Design review of the part built by this model. Coordinates are the model's own, in mm. A direction names the side the tool comes from. Give positions to 0.01 mm unless a question says otherwise; leave off trailing zeros. Write each loop counter-clockwise with the first axis right and the second up, starting at its lowest first coordinate (ties: lowest second). Pieces come first, ordered by that corner, then holes. Notation, with made-up numbers: (83, 62) -> (96, 62) arc R20 ccw to (96, 98) -> close; hole circle Ø7 at (20, -7). An arc over 180 degrees is marked (long way). Write each question's results on one line, items separated by ' | '. Start each with the question number.
(1) For faces 4 (the face through (25.186, -1.915, -4.619)), 5 (the face through (-7, 19, 10)), list the 3-axis set-ups (+Z, -Z, +X, -X, +Y, -Y) from which the entire face can be reached by the end or side of a thin tool; tool diameter is ignored.
(2) Take a section at A-A (x = 0). State the section outline as (y, z) points, plus the area to 3 significant figures.
(3) Mouldability with a two-part tool opening along Y and no side actions: class faces 1 (the face through (-4.336, -19.524, -0.14)), 2 (the face through (-2.994, 22.804, 0.14)), 3 (the face through (28, 0, 0)) as released by +Y, released by -Y, zero draft, split by the parting line, or undercut.
(4) Clearance check with flat-ended pins moving along their axes: pin 1 (3 mm diameter, centred on y = 17.5, z = 4, fed in from -X); pin 2 (5 mm diameter, centred on x = 1, z = 3.5, fed in from +Y); pin 3 (2 mm diameter, centred on x = -18, z = -4, fed in from +Y). State where each tip first meets the part, or that it passes through.
(5) Take a section at B-B (y = 0). State the section outline as (x, z) points.
(6) To check wall thickness, follow probe 1 along Y at (x, z) = (0, -1.5); probe 2 along X at (y, z) = (5.5, -5.25); probe 3 along X at (y, z) = (-7.5, -8). State the ranges of each line that lie inside material, in increasing order.
(7) Take a section at C-C (z = 0). State the section outline as (x, y) points, plus the area to 3 significant figures.
(8) Take a section at D-D (x = 8). State the section outline as (y, z) points, plus the area to 3 significant figures.
from build123d import *

# Parameters (mm, degrees)
ESQUISSE1_R                    = 23
ESQUISSE1_R_2                  = 20
BOSS_EXTRU_1_DEPTH             = 10
BOSS_EXTRU_2_REACH             = 48
ESQUISSE2_R                    = 5
BOSS_EXTRU_2_DIRECTION_2_DEPTH = 5


with BuildPart() as part:
    # Esquisse1 → Boss.-Extru.1 (new body, symmetric)
    with BuildSketch(Plane.XY):
        Circle(ESQUISSE1_R)
        Circle(ESQUISSE1_R_2, mode=Mode.SUBTRACT)
    extrude(amount=BOSS_EXTRU_1_DEPTH, both=True)

    # Esquisse2 → Boss.-Extru.2 (add, up to next)
    with BuildSketch(Plane(origin=(23, 0, 0), x_dir=(0, 0, -1), z_dir=(1, 0, 0)), mode=Mode.PRIVATE) as boss_extru_2_sk1:
        Circle(ESQUISSE2_R)
    boss_extru_2_tool1 = extrude(boss_extru_2_sk1.sketch, amount=-BOSS_EXTRU_2_REACH, mode=Mode.PRIVATE) - part.part
    add(boss_extru_2_tool1.solids().sort_by_distance((23, 0, 0))[0])
    add(boss_extru_2_tool1.solids().sort_by_distance((23, 0, 0))[1])

    # Esquisse2 → Boss.-Extru.2 direction 2 (add)
    with BuildSketch(Plane(origin=(23, 0, 0), x_dir=(0, 0, -1), z_dir=(1, 0, 0))):
        Circle(ESQUISSE2_R)
    extrude(amount=BOSS_EXTRU_2_DIRECTION_2_DEPTH)


solid = part.part
Report:
1) face 4: +X | face 5: +Z, +X, -X, +Y, -Y
2) outline: (-23, -10) -> (-20, -10) -> (-20, 10) -> (-23, 10) -> close; (20, -10) -> (23, -10) -> (23, 10) -> (20, 10) -> close | area: 120 mm2
3) face 1: undercut | face 2: split by the parting line | face 3: zero draft
4) pin 1: x = -16.52 | pin 2: y = 23 | pin 3: y = 15.49
5) outline: (-23, -10) -> (-20, -10) -> (-20, 10) -> (-23, 10) -> close; (20, -10) -> (23, -10) -> (23, -5) -> (28, -5) -> (28, 5) -> (23, 5) -> (23, 10) -> (20, 10) -> close
6) probe 1: -23 to -20, 20 to 23 | probe 2: -22.33 to -19.23, 19.23 to 22.33 | probe 3: -21.74 to -18.54, 18.54 to 21.74
7) outline: (22.45, -5) -> (28, -5) -> (28, 5) -> (22.45, 5) arc R23 ccw (long way) to start; hole circle Ø40 at (0, 0) | area: 457 mm2
8) outline: (-21.56, -10) -> (-18.33, -10) -> (-18.33, 10) -> (-21.56, 10) -> close; (18.33, -10) -> (21.56, -10) -> (21.56, 10) -> (18.33, 10) -> close | area: 129 mm2
